Autodesk Inventor part; units mm, degrees
ref_plane "Work Plane1" through (25, 0, 0) normal (0, 0, 1) x (1, 0, 0)
ref_plane "YZ Plane" through (0, 0, 0) normal (1, 0, 0) x (0, 1, 0)
ref_plane "XZ Plane" through (0, 0, 0) normal (0, 1, 0) x (-1, 0, 0)
sketch "Sketch1" plane through (0, 0, 0) normal (0, 0, 1) x (1, 0, 0)
  line L0 (-0.8667, 0) -> (61.25, 0)
  line L1 (61.25, 0) -> (61.25, 3)
  line L2 (61.25, 3) -> (50, 3)
  line L3 (50, 3) -> (50, 4)
  line L4 (50, 4) -> (0, 4)
  line L5 (0, 4) -> (0, 6.5)
  line L6 (0, 6.5) -> (-5.5, 6.5)
  line L7 (-5.5, 6.5) -> (-5.5, 2.3094)
  line L8 (-5.5, 2.3094) -> (-2.2, 2.3094)
  line L9 (-2.2, 2.3094) -> (-0.8667, 0)
  line L10 (-18.85, 0) -> (74.6, 0)
  line L11 (0, -1.3) -> (0, 7.8)
  line L12 (0, 3.71) -> (2.5, 3.71)
  line L13 (2.5, 3.71) -> (2.79, 4)
  line L14 (50, 3) -> (50, 2.3865)
  line L15 (50, 2.3865) -> (50.6135, 2.3865)
  line L16 (50.6135, 2.3865) -> (51.676, 3)
  line L17 (0, 3.71) -> (0, 4)
  dimension "d0" = 6
  dimension "d1" = 8
  dimension "d2" = 13
  dimension "d3" = 4.6188
  dimension "d5" = 11.25
  dimension "d6" = 5.5
  dimension "d7" = 3.3
  dimension "d8" = 60
  dimension "d9" = 61.25
  dimension "d18" = 2.5
  dimension "d19" = 45
  dimension "d20" = 7.42
  dimension "d21" = 4.7731
  dimension "d22" = 30
  dimension "d23" = 0.6135
revolve "Body" add sketch "Sketch1" angle 360 about axis through (-0.8667, 0, 0) along (1, 0, 0)
sketch "Sketch2" plane through (-5.5, 0, 0) normal (-1, 0, 0) x (0, 0, 1)
  circle A0 centre (0, 0) radius 2.3094
  line L0 (0, 2.3094) -> (2, 1.1547)
  line L1 (2, 1.1547) -> (2, -1.1547)
  line L2 (2, -1.1547) -> (0, -2.3094)
  line L3 (0, -2.3094) -> (-2, -1.1547)
  line L4 (-2, -1.1547) -> (-2, 1.1547)
  line L5 (-2, 1.1547) -> (0, 2.3094)
extrude "Slot" add sketch "Sketch2" against normal up to next contours A0 L1 | L0 A0 | A0 L2 | L5 A0 | A0 L3 | L4 A0
fillet "Fillet1" radius 2.3622 1 edges at (-5.5, -6.5, 0)
thread "Thread"
chamfer "Chamfer1" distance 0.6135 distance2 0.6135 1 edges at (61.25, -3, 0) measured on face at (61.25, 0.2734, 0.7208)
chamfer "Chamfer2" distance 0.15 angle 45 1 edges at (50, -4, 0)
revolve "Groove1" cut sketch "Sketch1" angle 360 about axis through (-0.8667, 0, 0) along (1, 0, 0) contours L11 L4 L13 L12
revolve "Groove2" cut sketch "Sketch1" angle 360 about axis through (-0.8667, 0, 0) along (1, 0, 0) contours L16 L15 L14 L2
ref_plane "Work Plane1" through (25, 0, 0) normal (0, 0, 1) x (1, 0, 0)
fillet "Fillet2" radius 0.4 1 edges at (50, -2.3865, 0)
fillet "Fillet3" radius 0.53 1 edges at (0, -3.71, 0)
equation "\"d0\" = NND"
equation "\"d1\" = BDM"
equation "\"d2\" = KOD"
equation "\"d3\" = 1.1547 * SW"
equation "\"d5\" = GEL"
equation "\"d6\" = KOH"
equation "\"d7\" = INTI + LOTI"
equation "\"d8\" = 0.5 * ANG"
equation "\"d9\" = NLG"
equation "\"d18\" = GAL2"
equation "\"d19\" = FAWI4"
equation "\"d20\" = BDMM"
equation "\"d21\" = GD1"
equation "\"d22\" = FAWI2"
equation "\"d23\" = GAL"
equation "\"d13\" = RR"
equation "\"d25\" = GEL"
equation "\"d14\" = -0.5 * SPD + 0.5 * NND"
equation "\"d15\" = GUL"
equation "\"d16\" = D1"
equation "\"d35\" = R1"
equation "\"d36\" = R2"
equation "\"NND\" = 6"
equation "\"NLG\" = 61.25"
equation "\"GEL\" = 11.25"
equation "\"KOD\" = 13"
equation "\"KOH\" = 5.5"
equation "\"INTI\" = 3.3"
equation "\"GAL\" = 0.61345 * PTC"
equation "\"GUL\" = 0.61345 * PTC"
equation "\"SPD\" = NND - 1.2269 * PTC"
equation "\"BDM\" = 8"
equation "\"ANG\" = 120deg"
equation "\"FAWI2\" = 30deg"
equation "\"FAWI3\" = 89deg"
equation "\"FAWI4\" = 45deg"
equation "\"RR\" = 2.3622"
equation "\"SW\" = 4"
equation "\"BDMM\" = 7.42"
equation "\"GAL2\" = 2.5"
equation "\"LOTI\" = 0"
equation "\"GD1\" = THREADDIA - 1.2269 * PTC"
equation "\"D1\" = 0.15"
equation "\"R1\" = 0.4"
equation "\"R2\" = 0.53"
equation "\"PTC\" = 1"
equation "\"BOR\" = 4"
equation "\"THREADDIA\" = 6"
equation "\"E0\" = 1.155 * SW"
equation "\"TOA\" = 30deg"
equation "\"PHH\" = 0.55"
properties part number "ISO  7379 - 8 x 50" material "Steel"
For this review, take the finished solid that the model builds, in its own axes (mm). A direction names the side the tool comes from. Coordinates: 2 decimals unless noted, no trailing zeros. Order: outer loops, then holes, each group sorted by start corner. A loop starts at its lowest first (then second) coordinate and runs counter-clockwise, first axis right, second up. Notation, with made-up numbers: (12.25, 13.25) - (50.25, 13.25) arc R20 cw to (50.25, 23.25) - close; hole circle Ø11 at (6.5, 79). An arc over 180 degrees is marked (long way). Answer as a JSON object with one key per item and string values. Group by question number.
1. Clearance check with flat-ended pins moving along their axes: P1, Ø5, axis at x = 44.5, y = 3.5, coming from the +Z side; P2, Ø4, axis at y = 2.5, z = 0.5, coming from the +X side; P3, Ø1.5, axis at x = 30, z = -2, coming from the +Y side; P4, Ø5, axis at x = 13, y = -1, coming from the +Z side. State where each tip first meets the part, or that it passes through.
2. For faces 4 (the cylindrical face through (56, -3, 0)), 5 (the flat face through (61.25, 0, 0)), 6 (the flat face through (-4, 0, 2)), list the 3-axis set-ups (+Z, -Z, +X, -X, +Y, -Y) from which the entire face can be reached by the end or side of a thin tool; tool diameter is ignored.
3. For probe 1 along X at (y, z) = (-3, 0.5); probe 2 along Z at (x, y) = (13.5, -1.5); probe 3 along Z at (x, y) = (14.5, 2.25), list the stretches that pass through material, from the lowest coordinate up.
4. We need section A-A on x = 16.5. State the section outline as (y, z) points, then the cut area to 3 significant figures.
5. The part is to be moulded in two halves that separate along Y. For faces 1 (the flat face through (50, 3, 1)), 2 (the cylindrical face through (25.991, -0.867, 3.905)), 3 (the flat face through (-4, 0, -2)), say which applies: pulls with the +Y half, pulls with the -Y half, needs draft (parallel to the pull), parting line crosses it, or undercut.
Final values:
{
 "1": {"P1": "z = 3.87", "P2": "x = 61.25", "P3": "y = 3.8", "P4": "z = 4"},
 "2": {"face 4": "+X", "face 5": "+Z, -Z, +X, +Y, -Y", "face 6": "-X"},
 "3": {"probe 1": "-5.5 to 50", "probe 2": "-3.71 to 3.71", "probe 3": "-3.31 to 3.31"},
 "4": {"outline": "circle Ø8 at (0, 0)", "area": "50.3 mm²"},
 "5": {"face 1": "needs draft", "face 2": "parting line crosses it", "face 3": "undercut"}
}
